Work out the finished part from the listing and answer in its coordinate system (mm). Give positions to 0.01 mm unless a question says otherwise; leave off trailing zeros. Order: outer loops, then holes, each group sorted by start corner. A loop starts at its lowest first (then second) coordinate and runs counter-clockwise, first axis right, second up. Notation, with made-up numbers: M 73,-20.5 L 107,-20.5 A26 cw 107,-4.5 Z; hole C 16.25,-2 d2. An arc over 180 degrees is marked long. One line per item, written item: value.
from build123d import *

# Parameters (mm, degrees)
MODEL_R             = 1.6
BOSS_EXTRUDE1_DEPTH = 1.5875


with BuildPart() as part:
    # Model → Boss-Extrude1 (new body)
    with BuildSketch(Plane.XY):
        with BuildLine():
            Line((127, 49.53), (127, 1.27))
            ThreePointArc((127, 1.27), (126.628025612, 0.371974388), (125.73, 0))
            Line((125.73, 0), (1.27, 0))
            ThreePointArc((1.27, 0), (0.371974388, 0.371974388), (0, 1.27))
            Line((0, 1.27), (0, 91.44))
            ThreePointArc((0, 91.44), (0.371974388, 92.338025612), (1.27, 92.71))
            Line((1.27, 92.71), (74.93, 92.71))
            ThreePointArc((74.93, 92.71), (75.828025612, 92.338025612), (76.2, 91.44))
            Line((76.2, 91.44), (76.2, 53.34))
            ThreePointArc((76.2, 53.34), (76.943948776, 51.543948776), (78.74, 50.8))
            Line((78.74, 50.8), (125.73, 50.8))
            ThreePointArc((125.73, 50.8), (126.628025612, 50.428025612), (127, 49.53))
        make_face()
        with Locations((2.54, 2.54)):
            Circle(MODEL_R, mode=Mode.SUBTRACT)
        with Locations((124.46, 2.54)):
            Circle(MODEL_R, mode=Mode.SUBTRACT)
        with Locations((2.54, 90.17)):
            Circle(MODEL_R, mode=Mode.SUBTRACT)
        with Locations((43.18, 2.54)):
            Circle(MODEL_R, mode=Mode.SUBTRACT)
        with Locations((83.82, 2.54)):
            Circle(MODEL_R, mode=Mode.SUBTRACT)
        with Locations((124.46, 48.26)):
            Circle(MODEL_R, mode=Mode.SUBTRACT)
        with Locations((73.66, 69.85)):
            Circle(MODEL_R, mode=Mode.SUBTRACT)
        with Locations((40.64, 69.85)):
            Circle(MODEL_R, mode=Mode.SUBTRACT)
        with Locations((40.64, 90.17)):
            Circle(MODEL_R, mode=Mode.SUBTRACT)
        with Locations((73.66, 90.17)):
            Circle(MODEL_R, mode=Mode.SUBTRACT)
    extrude(amount=-BOSS_EXTRUDE1_DEPTH)


solid = part.part
(1) Section B-B, the plane x = 83.82 is taken. Give the vertices of the cut face in (y, z), then the cut area to 3 significant figures.
Findings:
outline: M 0,-1.59 L 0.94,-1.59 L 0.94,0 L 0,0 Z; M 4.14,-1.59 L 50.8,-1.59 L 50.8,0 L 4.14,0 Z
area: 75.6 mm^2
(2) Section A-A, the plane y = 69.85 is taken. Give the vertices of the cut face in (x, z).
Findings:
outline: M 0,-1.59 L 39.04,-1.59 L 39.04,0 L 0,0 Z; M 42.24,-1.59 L 72.06,-1.59 L 72.06,0 L 42.24,0 Z; M 75.26,-1.59 L 76.2,-1.59 L 76.2,0 L 75.26,0 Z
(3) Determine the mould class of faces 1 (the cylindrical face through (2.19, 0.98, -0.78)), 2 (the cylindrical face through (76.924, 51.564, -0.783)), 3 (the flat face through (50, 37, 0)) for opening direction X: pulls with the +X half, pulls with the -X half, needs draft (parallel to the pull), parting line crosses it, or undercut.
Findings:
face 1: undercut
face 2: pulls with the +X half
face 3: needs draft
(4) Find the intervals of material crossed by probe 1 along X at (y, z) = (90.17, -0.85); probe 2 along Y at (x, z) = (2.54, -0.55); probe 3 along X at (y, z) = (69.85, -1.15), in increasing order. Write a range as from..to.
Findings:
probe 1: x = 0..0.94, 4.14..39.04, 42.24..72.06, 75.26..76.2
probe 2: y = 0..0.94, 4.14..88.57, 91.77..92.71
probe 3: x = 0..39.04, 42.24..72.06, 75.26..76.2
(5) Section C-C, the plane z = -0.9 is taken. Give the number of separate pieces and of enclosed holes in the cut face, then the cut area to 3 significant figures.
Findings:
separate pieces: 1
enclosed holes: 10
area: 9,560 mm^2
(6) Given P1, Ø0.8, axis at x = 97.5, z = -1, coming from the +Y side, flat-ended and moving along its own axis, determine where the tip first touches the part or whether it passes through.
Findings:
P1: stops at y = 50.8
(7) Section D-D, the plane y = 2.54 is taken. Give the vertices of the cut face in (x, z).
Findings:
outline: M 0,-1.59 L 0.94,-1.59 L 0.94,0 L 0,0 Z; M 4.14,-1.59 L 41.58,-1.59 L 41.58,0 L 4.14,0 Z; M 44.78,-1.59 L 82.22,-1.59 L 82.22,0 L 44.78,0 Z; M 85.42,-1.59 L 122.86,-1.59 L 122.86,0 L 85.42,0 Z; M 126.06,-1.59 L 127,-1.59 L 127,0 L 126.06,0 Z
